The listing builds one solid part. Answer for the finished solid, in the listing's coordinates (mm). A direction names the side the tool comes from. Give positions to 0.01 mm unless a question says otherwise; leave off trailing zeros. Order: outer loops, then holes, each group sorted by start corner. A loop starts at its lowest first (then second) coordinate and runs counter-clockwise, first axis right, second up. Notation, with made-up numbers: (-8.75, 12) - (-4.75, 12) arc R24 ccw to (-4.75, 43) - close; hole circle Ø4 at (68, 14). An arc over 180 degrees is marked (long way). Use a Markdown table: item, result. Add a question column.
1) Flat-ended cylindrical pins translate along their axes: pin 1 (1.8 mm diameter, centred on x = 33, z = -26.5, fed in from -Y); pin 2 (5.5 mm diameter, centred on x = 30.26, y = -50.5, fed in from -Z); pin 3 (3 mm diameter, centred on x = 38.5, z = -7, fed in from +Y); pin 4 (12.5 mm diameter, centred on x = 37.76, z = -10.01, fed in from -Y). Find the tip coordinate at first contact, or state that the pin passes through.
2) Find section D-D, the plane y = -18.5. Determine the outline of the cut face in (x, z).
3) For faces 4 (the face through (37, -50, -24.5)), 5 (the face through (35.5, -8, -25)), 6 (the face through (37, -44, 6)), 7 (the face through (46.7, -1.76, -25.04)), determine the directions among +Z, -Z, +X, -X, +Y, -Y from which every point of the face is accessible in a straight line to the end or side of a thin tool.
4) Find section B-B, the plane y = -8. Determine the outline of the cut face in (x, z), plus the area to 3 significant figures.
5) The mould has two halves that part along X. Classify faces 1 (the face through (25.12, -41.04, 7.1)), 2 (the face through (39.84, -7.19, -23.48)), 3 (the face through (37, -16, -22)): released by +X, released by -X, zero draft, split by the parting line, or undercut.
6) Straight lines are drawn through the part: line 1 (Z direction, x = 38, y = -53.5); line 2 (Z direction, x = 28.25, y = -3); line 3 (Y direction, x = 33.5, z = -3). For each, find the intervals that lie inside material, in ascending order.
7) Find section C-C, the plane z = -20.5. Determine the outline of the cut face in (x, y), plus the area to 3 significant figures.
8) Find section A-A, the plane y = -50.5. Determine the outline of the cut face in (x, z).
from build123d import *

# Parameters (mm, degrees)
BOSS_EXTRUDE1_DEPTH = 6
SKETCH2_W           = 26
SKETCH2_H           = 6
BOSS_EXTRUDE2_DEPTH = 40
FILLET1_R           = 12.5
SKETCH3_R           = 2.7
CUT_EXTRUDE1_DEPTH  = 7
SKETCH4_W           = 26
SKETCH4_H           = 29
BOSS_EXTRUDE3_DEPTH = 12
FILLET2_R           = 5
SKETCH5_R           = 1.75
CUT_EXTRUDE2_DEPTH  = 33.5
CUT_EXTRUDE3_DEPTH  = 41
CUT_EXTRUDE4_REACH  = 60
SKETCH7_R           = 5.4
FILLET3_R           = 2
SKETCH8_R           = 2.7
SKETCH8_R_2         = 1.6
BOSS_EXTRUDE4_DEPTH = 3


with BuildPart() as part:
    # Sketch1 → Boss-Extrude1 (new body)
    with BuildSketch(Plane(origin=(0, -44, 0), x_dir=(1, 0, 0), z_dir=(0, 1, 0))):
        with BuildLine():
            Line((50.264100782, -8), (50.264100782, 28))
            Line((50.264100782, 28), (27.264100782, 28))
            ThreePointArc((27.264100782, 28), (25.142780438, 27.121320344), (24.264100782, 25))
            Line((24.264100782, 25), (24.264100782, -5))
            ThreePointArc((24.264100782, -5), (25.142780438, -7.121320344), (27.264100782, -8))
            Line((27.264100782, -8), (50.264100782, -8))
        make_face()
    extrude(amount=BOSS_EXTRUDE1_DEPTH)

    # Sketch2 → Boss-Extrude2 (add)
    with BuildSketch(Plane(origin=(0, -38, 0), x_dir=(1, 0, 0), z_dir=(0, 1, 0))):
        with Locations((37.264100782, 25)):
            Rectangle(SKETCH2_W, SKETCH2_H)
    extrude(amount=BOSS_EXTRUDE2_DEPTH)

    # Fillet1
    fillet1_edges = [part.edges().sort_by_distance(p)[0] for p in [
        (50.264100782, 2, -25),
        (24.264100782, 2, -25),
    ]]
    fillet(fillet1_edges, radius=FILLET1_R)

    # Sketch3 → Cut-Extrude1 (cut, through all)
    with BuildSketch(Plane.XY.offset(-22)):
        with Locations((37.264100782, -8)):
            Circle(SKETCH3_R)
    extrude(amount=-CUT_EXTRUDE1_DEPTH, mode=Mode.SUBTRACT)

    # Sketch4 → Boss-Extrude3 (add)
    with BuildSketch(Plane.XZ.offset(44)):
        with Locations((37.264100782, -10)):
            Rectangle(SKETCH4_W, SKETCH4_H)
    extrude(amount=BOSS_EXTRUDE3_DEPTH)

    # Fillet2
    fillet2_edges = [part.edges().sort_by_distance(p)[0] for p in [
        (37.264100782, -38, -22),
    ]]
    fillet(fillet2_edges, radius=FILLET2_R)

    # Sketch5 → Cut-Extrude2 (cut, through all)
    with BuildSketch(Plane(origin=(0, 0, -24.5), x_dir=(-1, 0, 0), z_dir=(0, 0, -1))):
        with Locations((-45.264100782, -50.5)):
            Circle(SKETCH5_R)
        with Locations((-30.264100782, -50.5)):
            Circle(SKETCH5_R)
    extrude(amount=-CUT_EXTRUDE2_DEPTH, mode=Mode.SUBTRACT)

    # Sketch6 → Cut-Extrude3 (cut, through all)
    with BuildSketch(Plane.XZ.offset(38)):
        with BuildLine():
            Line((24.264100782, -28), (27.264100782, -28))
            ThreePointArc((27.264100782, -28), (25.142780438, -27.121320344), (24.264100782, -25))
            Line((24.264100782, -25), (24.264100782, -28))
        make_face()
    extrude(amount=-CUT_EXTRUDE3_DEPTH, mode=Mode.SUBTRACT)

    # Sketch7 → Cut-Extrude4 (cut, up to next)
    with BuildSketch(Plane.XZ.offset(56), mode=Mode.PRIVATE) as cut_extrude4_sk1:
        with Locations((37.764100782, -10.008379986)):
            Circle(SKETCH7_R)
    cut_extrude4_tool1 = extrude(cut_extrude4_sk1.sketch, amount=-CUT_EXTRUDE4_REACH, mode=Mode.PRIVATE) & part.part
    add(cut_extrude4_tool1.solids().sort_by_distance((37.764101, -56, -10.00838))[0], mode=Mode.SUBTRACT)

    # Fillet3
    fillet3_edges = [part.edges().sort_by_distance(p)[0] for p in [
        (32.364100782, -38, -10.008379986),
        (32.364100782, -56, -10.008379986),
    ]]
    fillet(fillet3_edges, radius=FILLET3_R)

    # Sketch8 → Boss-Extrude4 (add)
    with BuildSketch(Plane(origin=(0, 0, -28), x_dir=(-1, 0, 0), z_dir=(0, 0, -1))):
        with Locations((-37.264100782, -8)):
            Circle(SKETCH8_R)
        with Locations((-37.264100782, -8)):
            Circle(SKETCH8_R_2, mode=Mode.SUBTRACT)
    extrude(amount=-BOSS_EXTRUDE4_DEPTH)


solid = part.part
The answers:
| question | item | result |
|---|---|---|
| 1 | pin 1 | y = -44 |
| 1 | pin 2 | z = -24.5 |
| 1 | pin 3 | through |
| 1 | pin 4 | y = -55.64 |
| 2 | outline | (24.26, -25) arc R3 ccw to (27.26, -28) - (50.26, -28) - (50.26, -22) - (24.26, -22) - close |
| 3 | face 4 | -Z, +X, -X, -Y |
| 3 | face 5 | +Z |
| 3 | face 6 | +Z, +X, -X, -Y |
| 3 | face 7 | +Z, -Z, +X, +Y |
| 4 | outline | (24.52, -26.2) arc R3 ccw to (27.26, -28) - (35.66, -28) - (35.66, -25) - (34.56, -25) - (34.56, -22) - (24.52, -22) - close; (38.86, -28) - (50.01, -28) - (50.01, -22) - (39.96, -22) - (39.96, -25) - (38.86, -25) - close |
| 4 | area | 126 mm2 |
| 5 | face 1 | released by -X |
| 5 | face 2 | undercut |
| 5 | face 3 | zero draft |
| 6 | line 1 | -24.5 to -15.4, -4.61 to 4.5 |
| 6 | line 2 | -28 to -22 |
| 6 | line 3 | -56 to -38 |
| 7 | outline | (24.26, -56) - (50.26, -56) - (50.26, -36.57) - (24.26, -36.57) - close; hole circle Ø3.5 at (30.26, -50.5); hole circle Ø3.5 at (45.26, -50.5) |
| 7 | area | 486 mm2 |
| 8 | outline | (24.26, -24.5) - (28.51, -24.5) - (28.51, 4.5) - (24.26, 4.5) - close; (32.01, -24.5) - (43.51, -24.5) - (43.51, 4.5) - (32.01, 4.5) - close; (47.01, -24.5) - (50.26, -24.5) - (50.26, 4.5) - (47.01, 4.5) - close; hole circle Ø10.8 at (37.76, -10.01) |
